from build123d import *

# Parameters (mm, degrees)
SKETCH2_W           = 12
SKETCH2_H           = 22
BOSS_EXTRUDE1_DEPTH = 22
SKETCH4_W           = 8
SKETCH4_H           = 20
CUT_EXTRUDE1_DEPTH  = 18
CUT_EXTRUDE2_DEPTH  = 10


with BuildPart() as part:
    # Sketch2 → Boss-Extrude1 (new body)
    with BuildSketch(Plane(origin=(0, 0, 0), x_dir=(1, 0, 0), z_dir=(0, 1, 0))):
        with Locations((6, 11)):
            Rectangle(SKETCH2_W, SKETCH2_H)
    extrude(amount=BOSS_EXTRUDE1_DEPTH)

    # Sketch4 → Cut-Extrude1 (cut)
    with BuildSketch(Plane.XY):
        with Locations((6, 10.85774702)):
            Rectangle(SKETCH4_W, SKETCH4_H)
    extrude(amount=-CUT_EXTRUDE1_DEPTH, mode=Mode.SUBTRACT)

    # Sketch6 → Cut-Extrude2 (cut)
    with BuildSketch(Plane.XY.offset(-18)):
        with BuildLine():
            Line((5, 2.55774702), (5, 19.15774702))
            ThreePointArc((5, 19.15774702), (6, 20.15774702), (7, 19.15774702))
            Line((7, 19.15774702), (7, 2.55774702))
            ThreePointArc((7, 2.55774702), (6, 1.55774702), (5, 2.55774702))
        make_face()
    extrude(amount=-CUT_EXTRUDE2_DEPTH, mode=Mode.SUBTRACT)


solid = part.part
Read the model definition and answer for the solid it produces. Units are mm, in the model's axes. A direction names the side the tool comes from. Coordinates: 2 decimals unless noted, no trailing zeros. Loops run counter-clockwise (first coordinate to the right, second up) from the corner with the lowest first, then second, coordinate; pieces in that order, holes last. Notation, with made-up numbers: (64.5, 14) - (79.5, 14) arc R24 ccw to (79.5, 45) - close; hole circle Ø5 at (43.5, 83.5). An arc over 180 degrees is marked (long way). Answer in a Markdown table with one row per item.
Q1. The mould has two halves that part along X. Classify faces 1 (the flat face through (0, 11, -11)), 2 (the flat face through (4.6, 10.8, -22)), 3 (the cylindrical face through (6.022, 1.558, -19.972)): pulls with the +X half, pulls with the -X half, needs draft (parallel to the pull), parting line crosses it, or undercut.
Here are the results:
| item | result |
|---|---|
| face 1 | pulls with the -X half |
| face 2 | needs draft |
| face 3 | undercut |
Q2. Find section C-C on x = 6. Write down the section's boundary in (y, z).
Here are the results:
| item | result |
|---|---|
| outline | (0, -22) - (1.56, -22) - (1.56, -18) - (0.86, -18) - (0.86, 0) - (0, 0) - close; (20.16, -22) - (22, -22) - (22, 0) - (20.86, 0) - (20.86, -18) - (20.16, -18) - close |
Q3. Find section D-D on x = 2.75. Write down the section's boundary in (y, z), plus the area to 3 significant figures.
Here are the results:
| item | result |
|---|---|
| outline | (0, -22) - (22, -22) - (22, 0) - (20.86, 0) - (20.86, -18) - (0.86, -18) - (0.86, 0) - (0, 0) - close |
| area | 124 mm^2 |
Q4. For faces 4 (the flat face through (12, 11, -11)), 5 (the flat face through (6, 20.858, -9)), 6 (the flat face through (7, 11, -20)), determine the directions among +Z, -Z, +X, -X, +Y, -Y from which every point of the face is accessible in a straight line to the end or side of a thin tool.
Here are the results:
| item | result |
|---|---|
| face 4 | +Z, -Z, +X, +Y, -Y |
| face 5 | +Z |
| face 6 | +Z, -Z |
Q5. Find section B-B on z = -17.5. Write down the section's boundary in (x, y).
Here are the results:
| item | result |
|---|---|
| outline | (0, 0) - (12, 0) - (12, 22) - (0, 22) - close; hole (2, 0.86) - (10, 0.86) - (10, 20.86) - (2, 20.86) - close |
Q6. Find section A-A on y = 13.75. Write down the section's boundary in (x, z), plus the area to 3 significant figures.
Here are the results:
| item | result |
|---|---|
| outline | (0, -22) - (5, -22) - (5, -18) - (2, -18) - (2, 0) - (0, 0) - close; (7, -22) - (12, -22) - (12, 0) - (10, 0) - (10, -18) - (7, -18) - close |
| area | 112 mm^2 |
Q7. Straight lines are drawn through the part: line 1 along X through (y, z) = (1.5, -4.5); line 2 along Y through (x, z) = (8.75, -10.75); line 3 along X through (y, z) = (3.25, -19.75). For each, find the intervals that lie inside material, in ascending order. Write a range as [from, to].
Here are the results:
| item | result |
|---|---|
| line 1 | x = [0, 2], [10, 12] |
| line 2 | y = [0, 0.86], [20.86, 22] |
| line 3 | x = [0, 5], [7, 12] |
